Input: part model. Units: mm. Frame: model coordinates. Give positions to 0.01 mm unless a question says otherwise; leave off trailing zeros. Loops run counter-clockwise (first coordinate to the right, second up) from the corner with the lowest first, then second, coordinate; pieces in that order, holes last. Notation, with made-up numbers: (75.25, 43) -> (111.25, 43) arc R25 ccw to (111.25, 59) -> close; hole circle Ø7 at (80.5, 55). An arc over 180 degrees is marked (long way). Answer as a JSON object with one key per item and string values. Group by question number.
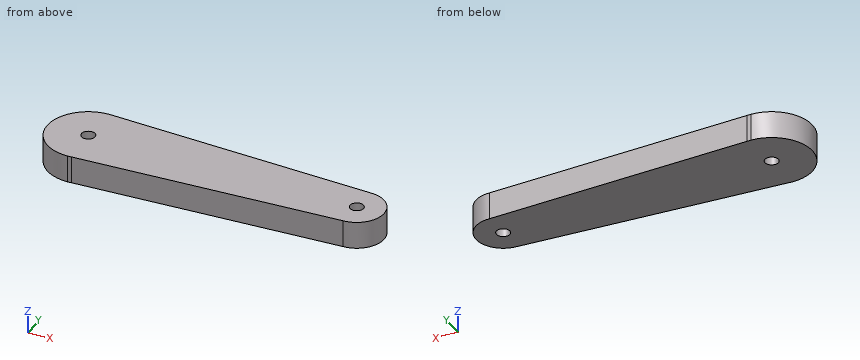
```python
from build123d import *

# Parameters (mm, degrees)
SKETCH1_R           = 10
BOSS_EXTRUDE1_DEPTH = 10
SKETCH9_R           = 2.5
CUT_EXTRUDE7_DEPTH  = 10


with BuildPart() as part:
    # Sketch1 → Boss-Extrude1 (new body)
    with BuildSketch(Plane.XY):
        with BuildLine():
            Line((-36.34910837, 14.107005992), (-37.845367722, 14.18181896))
            ThreePointArc((-37.845367722, 14.18181896), (-52.845367722, -0.81818104), (-37.845367722, -15.81818104))
            Line((-37.845367722, -15.81818104), (-36.34910837, -15.743368072))
            ThreePointArc((-36.34910837, -15.743368072), (-26.722331035, -10.8818809), (-22.845367722, -0.81818104))
            ThreePointArc((-22.845367722, -0.81818104), (-26.722331035, 9.245518819), (-36.34910837, 14.107005992))
        make_face()
        with BuildLine():
            Line((62.154632278, 9.18181896), (-36.34910837, 14.107005992))
            ThreePointArc((-36.34910837, 14.107005992), (-26.722331035, 9.245518819), (-22.845367722, -0.81818104))
            ThreePointArc((-22.845367722, -0.81818104), (-26.722331035, -10.8818809), (-36.34910837, -15.743368072))
            Line((-36.34910837, -15.743368072), (62.154632278, -10.81818104))
            ThreePointArc((62.154632278, -10.81818104), (52.154632278, -0.81818104), (62.154632278, 9.18181896))
        make_face()
        with Locations((62.154632278, -0.81818104)):
            Circle(SKETCH1_R)
    extrude(amount=BOSS_EXTRUDE1_DEPTH)

    # Sketch9 → Cut-Extrude7 (cut)
    with BuildSketch(Plane.XY.offset(10)):
        with Locations((-37.845367722, -0.81818104)):
            Circle(SKETCH9_R)
        with Locations((62.154632278, -0.81818104)):
            Circle(SKETCH9_R)
    extrude(amount=-CUT_EXTRUDE7_DEPTH, mode=Mode.SUBTRACT)


solid = part.part
```
Q1. Pin query (flat end, axial travel): pin 1 Ø4 at (y, z) = (9, 1.5) entering from -X; pin 2 Ø2 at (y, z) = (-7, 7) entering from -X; pin 3 Ø1 at (x, z) = (-24.5, 5.5) entering from +Y. Return the tip coordinate at first contact, or that it passes through.
Q2. Section B-B on z = 3. Return the cut outline in (x, y).
Q3. Section A-A on x = 61. Return the cut outline in (y, z).
Q4. Section C-C on y = 5.75. Return the cut outline in (x, z), then the cut area to 3 significant figures.
Q5. Ray query, probe 1 along X at (y, z) = (-2.5, 0.75); probe 2 along Y at (x, z) = (-36.5, 9); probe 3 along X at (y, z) = (-9.75, 3). Return the intervals inside material, ascending.
Q6. Section D-D on x = -31. Return the cut outline in (y, z).
Numbers:
{
 "1": {"pin 1": "stops at x = -50.65", "pin 2": "stops at x = -51.92", "pin 3": "stops at y = 13.54"},
 "2": {"outline": "(-37.85, -15.82) -> (62.15, -10.82) arc R10 ccw to (62.15, 9.18) -> (-37.85, 14.18) arc R15 ccw to start; hole circle Ø5 at (-37.85, -0.82); hole circle Ø5 at (62.15, -0.82)"},
 "3": {"outline": "(-10.88, 0) -> (-3.04, 0) -> (-3.04, 10) -> (-10.88, 10) -> close; (1.4, 0) -> (9.24, 0) -> (9.24, 10) -> (1.4, 10) -> close"},
 "4": {"outline": "(-51.33, 0) -> (69.7, 0) -> (69.7, 10) -> (-51.33, 10) -> close", "area": "1,210 mm²"},
 "5": {"probe 1": "x = -52.75 to -39.7, -36 to 60.3, 64 to 72.01", "probe 2": "y = -15.75 to -2.93, 1.29 to 14.11", "probe 3": "x = -49.9 to 66.65"},
 "6": {"outline": "(-15.48, 0) -> (13.84, 0) -> (13.84, 10) -> (-15.48, 10) -> close"}
}
